Source: three-view drawing plus pictorial views. Frame: mm from the lowest corner of the part. A direction names the side the tool comes from. Round coordinates to 2 decimals unless told otherwise and drop trailing zeros. Write each loop counter-clockwise with the first axis right and the second up, starting at its lowest first coordinate (ties: lowest second). Pieces come first, ordered by that corner, then holes. Notation, with made-up numbers: M 22,46.25 L 61,46.25 A27 cw 61,85.25 Z; hole C 63,-31 d3. An arc over 180 degrees is marked long. Answer as CSV lines item,"result". Start each with the question number.
Q1. First-contact query: pin 1 (1.5 mm diameter, centred on x = 3, z = 1.5, fed in from +Y); pin 2 (1.5 mm diameter, centred on y = 2.5, z = 2, fed in from -X); pin 3 (1 mm diameter, centred on y = 2, z = 1.5, fed in from +X). Flat tips, straight axial feed; report the tip coordinate or a pass-through.
Q2. Section query B-B on z = 3. Output: boundary loops of the cut face in (x, y).
Q3. Mould query, pull axis X, two halves, no side actions, for the marked faces 3, 4 and 5. Classes: pulls with the +X half, pulls with the -X half, needs draft (parallel to the pull), parting line crosses it, or undercut.
Q4. Ray query, probe 1 along Y at (x, z) = (1.9, 3.25); probe 2 along Z at (x, y) = (2.35, 1.55); probe 3 along Z at (x, y) = (3.2, 0.9). Return the intervals inside material, ascending.
Q5. Section query A-A on z = 8.75. Output: boundary loops of the cut face in (x, y), and give its area (3 significant figures).
Q6. Reachability of the marked faces 1 and 2 from +Z, -Z, +X, -X, +Y, -Y: full face, straight path, thin tool, end or side. Return the list, or none.
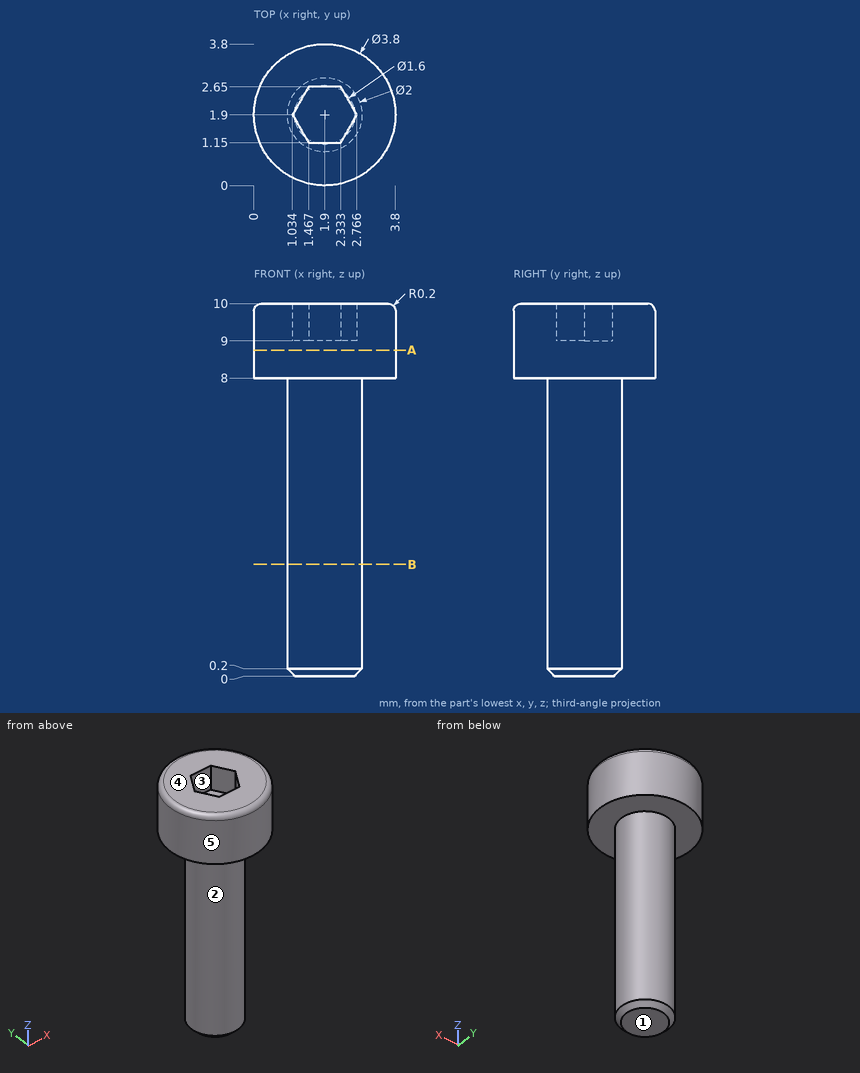
Entries:
1,pin 1,"stops at y = 2.84"
1,pin 2,"stops at x = 0.9"
1,pin 3,"stops at x = 2.9"
2,outline,"C 1.9,1.9 d2"
3,face 3,"undercut"
3,face 4,"needs draft"
3,face 5,"parting line crosses it"
4,probe 1,"y = 0.9 to 2.9"
4,probe 2,"z = 0 to 9"
4,probe 3,"z = 8 to 10"
5,outline,"C 1.9,1.9 d3.8"
5,area,"11.3 mm^2"
6,face 1,"-Z, +X, -X, +Y, -Y"
6,face 2,"-Z"
